Verification items for the finished model (mm, model axes). Round coordinates to 2 decimals unless told otherwise and drop trailing zeros. Write each loop counter-clockwise with the first axis right and the second up, starting at its lowest first coordinate (ties: lowest second). Pieces come first, ordered by that corner, then holes. Notation, with made-up numbers: (77, 50) -> (117, 50) arc R4 cw to (117, 55) -> close; hole circle Ø8 at (1.5, 46.5). An arc over 180 degrees is marked (long way). Answer as a JSON object with one key per item and string values. Group by question number.
(1) Sectioned sample at A-A on z = 38. Record the cut outline in (x, y), and give its area (3 significant figures).
(2) Gauge pin test, flat end, axial feed: pin 1 Ø6 at (x, y) = (-24, 3.5) entering from -Z. Record the tip position at first contact, or that the pin passes through.
(3) Draft check along Y on faces 1 (the face through (-29.3, 18.6, 41.6)), 2 (the face through (0, -19, 42)), 3 (the face through (-3.347, 0.147, 36.468)). Enter one of: released by +Y, released by -Y, zero draft, split by the parting line, or undercut.
(4) Sectioned sample at C-C on x = 0. Record the cut outline in (y, z).
(5) Sectioned sample at B-B on y = 0. Record the cut outline in (x, z).
(6) Scan lines: L1, parallel to Y at x = 0, z = 38.25; L2, parallel to X at y = 15.5, z = 35; L3, parallel to X at y = 14, z = 32.75. Record each from-to range of solid material in increasing order. Write a range as from..to.
(7) Sectioned sample at D-D on y = -4. Record the cut outline in (x, z), and give its area (3 significant figures).
```python
from build123d import *

# Parameters (mm, degrees)
SKETCH002_W             = 61
SKETCH002_H             = 40
PAD001_DEPTH            = 13.25
POCKET_DEPTH            = 40
SKETCH007_R             = 3.35
POCKET001_DEPTH         = 13.25
CHAMFER_SIZE            = 2
BODY002_PLACEMENT_ANGLE = 180


with BuildPart() as part:
    # Sketch002 → Pad001 (new body)
    with BuildSketch(Plane.XY):
        Rectangle(SKETCH002_W, SKETCH002_H)
    extrude(amount=PAD001_DEPTH)

    # Sketch003 (on Face3 of Pad001) → Pocket (cut)
    with BuildSketch(Plane.XZ.offset(20)):
        with BuildLine():
            ThreePointArc((-25.5, 14.25), (-15.25, 4), (-5, 14.25))
            Line((-25.5, 14.25), (-5, 14.25))
        make_face()
        with BuildLine():
            ThreePointArc((5, 14.25), (15.25, 4), (25.5, 14.25))
            Line((5, 14.25), (25.5, 14.25))
        make_face()
    extrude(amount=-POCKET_DEPTH, mode=Mode.SUBTRACT)


with BuildPart() as part_1:
    # Body001 placement: moved
    add(part.part.moved(Location((0, 0, 7))))

    # Sketch007 (on DatumPlane) → Pocket001 (cut)
    with BuildSketch(Plane(origin=(0, 0, 7), x_dir=(1, 0, 0), z_dir=(0, 0, -1))):
        Circle(SKETCH007_R)
    extrude(amount=-POCKET001_DEPTH, mode=Mode.SUBTRACT)

    # Chamfer
    chamfer_edges = [part_1.edges().sort_by_distance(p)[0] for p in [
        (30.5, 0, 7),
        (0, -20, 7),
        (-30.5, 0, 7),
        (0, 20, 7),
        (30.5, -20, 13.625),
        (30.5, 20, 13.625),
        (-30.5, 20, 13.625),
        (-30.5, -20, 13.625),
    ]]
    chamfer(chamfer_edges, length=CHAMFER_SIZE)


with BuildPart() as part_2:
    # Body002 placement: moved
    add(part_1.part.moved(Location((0, 0, 50))).rotate(Axis((0, 0, 50), (1, 0, 0)), BODY002_PLACEMENT_ANGLE))


solid = part_2.part
```
Computed values:
{
 "1": {"outline": "(-30.5, -18) -> (-28.5, -20) -> (-19.67, -20) -> (-19.67, 20) -> (-28.5, 20) -> (-30.5, 18) -> close; (-10.83, -20) -> (10.83, -20) -> (10.83, 20) -> (-10.83, 20) -> close; (19.67, -20) -> (28.5, -20) -> (30.5, -18) -> (30.5, 18) -> (28.5, 20) -> (19.67, 20) -> close; hole circle Ø6.7 at (0, 0)", "area": "1,690 mm2"},
 "2": {"pin 1": "z = 29.75"},
 "3": {"face 1": "released by +Y", "face 2": "released by -Y", "face 3": "undercut"},
 "4": {"outline": "(-20, 29.75) -> (-3.35, 29.75) -> (-3.35, 43) -> (-18, 43) -> (-20, 41) -> close; (3.35, 29.75) -> (20, 29.75) -> (20, 41) -> (18, 43) -> (3.35, 43) -> close"},
 "5": {"outline": "(-30.5, 29.75) -> (-25.45, 29.75) arc R10.25 cw to (-5.05, 29.75) -> (-3.35, 29.75) -> (-3.35, 43) -> (-28.5, 43) -> (-30.5, 41) -> close; (3.35, 29.75) -> (5.05, 29.75) arc R10.25 cw to (25.45, 29.75) -> (30.5, 29.75) -> (30.5, 41) -> (28.5, 43) -> (3.35, 43) -> close"},
 "6": {"L1": "-20..-3.35, 3.35..20", "L2": "-30.5..-23.37, -7.13..7.13, 23.37..30.5", "L3": "-30.5..-24.69, -5.81..5.81, 24.69..30.5"},
 "7": {"outline": "(-30.5, 29.75) -> (-25.45, 29.75) arc R10.25 cw to (-5.05, 29.75) -> (5.05, 29.75) arc R10.25 cw to (25.45, 29.75) -> (30.5, 29.75) -> (30.5, 41) -> (28.5, 43) -> (-28.5, 43) -> (-30.5, 41) -> close", "area": "515 mm2"}
}
